Geometry: final body of the model. Coordinates: model frame, mm. A direction names the side the tool comes from. Give positions to 0.01 mm unless a question says otherwise; leave off trailing zeros. Loops run counter-clockwise (first coordinate to the right, second up) from the corner with the lowest first, then second, coordinate; pieces in that order, holes last.
1. Draft query along Y for faces 1 (the face through (38, 12, 1.016)), 2 (the face through (38, 22, 11.336)), 3 (the face through (38, 0, 6)). Return one class per face: +Y half, -Y half, draft (parallel to the pull), parting line (faces both ways), or undercut.
2. Material intervals for line 1 along X through (y, z) = (16.5, 4.5); line 2 along Y through (x, z) = (66.5, 8); line 3 along Z through (x, y) = (62, 18.5), sorted ascending.
3. Access query for faces 4 (the face through (77, 11, 10)), 5 (the face through (38, 20.86, 7)), 6 (the face through (1.8, 15.68, 3.9)), 7 (the face through (38, 1, 11.336)). Directions: +Z, -Z, +X, -X, +Y, -Y. A direction counts if a zero-diameter tool reaches every point of the face in a straight line with its end or side. Return the directions, or none.
4. First-contact query: P1, Ø0.8, axis at y = 13.5, z = 0.5, coming from the +X side; P2, Ø2, axis at x = 76.5, y = 13, coming from the -Z side; P3, Ø1.1, axis at y = 13.5, z = 0.5, coming from the -X side. Flat tips, straight axial feed; report the tip coordinate or a pass-through.
5. Section D-D, the plane x = 23. Output: boundary loops of the cut face in (y, z), then the cut area to 3 significant figures.
6. Section C-C, the plane y = 6.5. Output: boundary loops of the cut face in (x, z), then the cut area to 3 significant figures.
7. Section B-B, the plane y = 13. Output: boundary loops of the cut face in (x, z), then the cut area to 3 significant figures.
8. Section A-A, the plane z = 8.75. Output: boundary loops of the cut face in (x, y).
from build123d import *

# Parameters (mm, degrees)
F0_W          = 77.724
F0_H          = 22.86
F1_DEPTH      = 21.336
F2_W          = 73.724
F2_H          = 18.86
F3_DEPTH      = 20.32
F4_W          = 7.62
F4_H          = 8.5
F5_DEPTH      = 10
F6_W          = 73.724
F6_H          = 10
F7_DEPTH      = 25
F7_DEPTH_BACK = 25
F8_T1_DEPTH   = 2
F8_T3_DEPTH   = 2
F8_T8_DEPTH   = 52.7937003968
F8_T14_DEPTH  = 52.7937003968
F8_T20_DEPTH  = 52.7937003968
F8_T26_DEPTH  = 52.7937003968


# Not quite as in the source:
# - a fillet or chamfer that OpenCascade refuses, or shapes differently, is made with other operations: its cross-section is extruded or revolved along the edge and cut away or added


with BuildPart() as f1:
    # F0 (on Top) → F1 (new body)
    with BuildSketch(Plane.XY):
        with Locations((38.862, 11.43)):
            Rectangle(F0_W, F0_H)
    extrude(amount=F1_DEPTH)

    # F2 (on face) → F3 (cut)
    with BuildSketch(Plane.XY.offset(21.336)):
        with Locations((38.862, 11.43)):
            Rectangle(F2_W, F2_H)
    extrude(amount=-F3_DEPTH, mode=Mode.SUBTRACT)

    # F4 (on face) → F5 (cut)
    with BuildSketch(Plane(origin=(0, 0, 0), x_dir=(1, 0, 0), z_dir=(0, 0, -1))):
        with Locations((3.81, -11.43)):
            Rectangle(F4_W, F4_H)
        with Locations((73.914, -11.43)):
            Rectangle(F4_W, F4_H)
    extrude(amount=-F5_DEPTH, mode=Mode.SUBTRACT)

    # F6 (on Front) → F7 (cut, two sides)
    with BuildSketch(Plane.XZ) as f7_sk:
        with Locations((38.862, 16.336)):
            Rectangle(F6_W, F6_H)
    extrude(amount=-F7_DEPTH, mode=Mode.SUBTRACT)
    extrude(f7_sk.sketch, amount=F7_DEPTH_BACK, mode=Mode.SUBTRACT)

    # F8: fillet of radius 10.16 on 4 edges, made by hand

    # F8_s2 → F8_t1 (join)
    with BuildSketch(Plane.XZ.offset(-2)):
        with BuildLine():
            ThreePointArc((12.1587400794, 11.336), (5.0313282069, 14.2554475349), (2, 21.336))
            Line((2, 21.336), (2, 11.336))
            Line((2, 11.336), (12.1587400794, 11.336))
        make_face()
        with BuildLine():
            ThreePointArc((65.5652599206, 11.336), (72.6926717931, 14.2554475349), (75.724, 21.336))
            Line((75.724, 21.336), (75.724, 11.336))
            Line((75.724, 11.336), (65.5652599206, 11.336))
        make_face()
    extrude(amount=F8_T1_DEPTH)

    # F8_s4 → F8_t3 (join)
    with BuildSketch(Plane.XZ.offset(-22.86)):
        with BuildLine():
            ThreePointArc((12.1587400794, 11.336), (5.0313282069, 14.2554475349), (2, 21.336))
            Line((2, 21.336), (2, 11.336))
            Line((2, 11.336), (12.1587400794, 11.336))
        make_face()
        with BuildLine():
            ThreePointArc((75.724, 21.336), (72.6926717931, 14.2554475349), (65.5652599206, 11.336))
            Line((65.5652599206, 11.336), (75.724, 11.336))
            Line((75.724, 11.336), (75.724, 21.336))
        make_face()
    extrude(amount=F8_T3_DEPTH)


with BuildPart() as f8_tool6:
    # F8_s7 → F8_t8 (new body)
    with BuildSketch(Plane.XZ.offset(-27.3968501984)):
        with BuildLine():
            ThreePointArc((12.1587400794, 11.336), (5.0313282069, 14.2554475349), (2, 21.336))
            Line((2, 21.336), (2, 11.336))
            Line((2, 11.336), (12.1587400794, 11.336))
        make_face()
    extrude(amount=F8_T8_DEPTH)

    split(bisect_by=Plane.XZ.offset(-22.86), keep=Keep.TOP)

    split(bisect_by=Plane.XZ.offset(-20.86), keep=Keep.BOTTOM)


with BuildPart() as f1_1:
    add(f1.part)

    # F8_t5: union F8_tool6
    add(f8_tool6.part)


with BuildPart() as f8_tool12:
    # F8_s13 → F8_t14 (new body)
    with BuildSketch(Plane.XZ.offset(-48.2568501984)):
        with BuildLine():
            ThreePointArc((12.1587400794, 11.336), (5.0313282069, 14.2554475349), (2, 21.336))
            Line((2, 21.336), (2, 11.336))
            Line((2, 11.336), (12.1587400794, 11.336))
        make_face()
    extrude(amount=F8_T14_DEPTH)

    split(bisect_by=Plane.XZ.offset(-2), keep=Keep.TOP)

    split(bisect_by=Plane.XZ, keep=Keep.BOTTOM)


with BuildPart() as f1_2:
    add(f1_1.part)

    # F8_t11: union F8_tool12
    add(f8_tool12.part)


with BuildPart() as f8_tool18:
    # F8_s19 → F8_t20 (new body)
    with BuildSketch(Plane.XZ.offset(25.3968501984)):
        with BuildLine():
            ThreePointArc((65.5652599206, 11.336), (72.6926717931, 14.2554475349), (75.724, 21.336))
            Line((75.724, 21.336), (75.724, 11.336))
            Line((75.724, 11.336), (65.5652599206, 11.336))
        make_face()
    extrude(amount=-F8_T20_DEPTH)

    split(bisect_by=Plane.XZ.offset(-22.86), keep=Keep.TOP)

    split(bisect_by=Plane.XZ.offset(-20.86), keep=Keep.BOTTOM)


with BuildPart() as f1_3:
    add(f1_2.part)

    # F8_t17: union F8_tool18
    add(f8_tool18.part)


with BuildPart() as f8_tool24:
    # F8_s25 → F8_t26 (new body)
    with BuildSketch(Plane.XZ.offset(4.5368501984)):
        with BuildLine():
            ThreePointArc((75.724, 21.336), (72.6926717931, 14.2554475349), (65.5652599206, 11.336))
            Line((65.5652599206, 11.336), (75.724, 11.336))
            Line((75.724, 11.336), (75.724, 21.336))
        make_face()
    extrude(amount=-F8_T26_DEPTH)

    split(bisect_by=Plane.XZ.offset(-2), keep=Keep.TOP)

    split(bisect_by=Plane.XZ, keep=Keep.BOTTOM)


with BuildPart() as f1_4:
    add(f1_3.part)

    # F8_t23: union F8_tool24
    add(f8_tool24.part)


solid = f1_4.part
Answers below:
1. face 1: undercut
1. face 2: draft
1. face 3: -Y half
2. line 1: x = 0 to 2, 75.72 to 77.72
2. line 2: y = 0 to 2, 20.86 to 22.86
2. line 3: z = 0 to 1.02
3. face 4: -Z, +X, -X
3. face 5: +Z
3. face 6: -Z, -X
3. face 7: +Z, +Y, -Y
4. P1: stops at x = 70.1
4. P2: stops at z = 10
4. P3: stops at x = 7.62
5. outline: (0, 0) - (22.86, 0) - (22.86, 11.34) - (20.86, 11.34) - (20.86, 1.02) - (2, 1.02) - (2, 11.34) - (0, 11.34) - close
5. area: 64.5 mm2
6. outline: (0, 0) - (77.72, 0) - (77.72, 21.34) - (75.72, 21.34) - (75.72, 1.02) - (2, 1.02) - (2, 21.34) - (0, 21.34) - close
6. area: 160 mm2
7. outline: (0, 10) - (2, 10) - (2, 21.34) - (0, 21.34) - close; (7.62, 0) - (70.1, 0) - (70.1, 1.02) - (7.62, 1.02) - close; (75.72, 10) - (77.72, 10) - (77.72, 21.34) - (75.72, 21.34) - close
7. area: 109 mm2
8. outline: (0, 0) - (77.72, 0) - (77.72, 7.18) - (75.72, 7.18) - (75.72, 2) - (2, 2) - (2, 7.18) - (0, 7.18) - close; (0, 15.68) - (2, 15.68) - (2, 20.86) - (75.72, 20.86) - (75.72, 15.68) - (77.72, 15.68) - (77.72, 22.86) - (0, 22.86) - close
